Check sheet for the modelled part. Datum: model origin and axes. Units: mm. A direction names the side the tool comes from. Round coordinates to 2 decimals unless told otherwise and drop trailing zeros. Loops run counter-clockwise (first coordinate to the right, second up) from the corner with the lowest first, then second, coordinate; pieces in that order, holes last. Notation, with made-up numbers: (29, 54.25) -> (50, 54.25) arc R22 cw to (50, 77.25) -> close; hole circle Ø11 at (83.5, -28). An arc over 180 degrees is marked (long way). One line per item, written item: value. Start each with the question number.
1. Cross-section at C-C on z = 110. Record the cut outline in (x, y).
2. Go/stop test with flat-tipped pins: pin 1 (3 mm diameter, centred on x = -3, z = 37.5, fed in from +Y); pin 2 (8.5 mm diameter, centred on x = 2, z = 107.5, fed in from -Y); pin 3 (2 mm diameter, centred on x = -2, z = 102.5, fed in from +Y); pin 4 (13.5 mm diameter, centred on x = 0, y = 0, fed in from +Z). Record where each tip stops, or that it passes through.
3. Cross-section at A-A on y = 0. Record the cut outline in (x, z), then the cut area to 3 significant figures.
4. Release check for a two-part mould opening along Y. For faces 4 (the face through (12.114, 3.815, 108.46)), 5 (the face through (0, 11.5, 102)), 6 (the face through (2, -11.5, 108)), 7 (the face through (-2.395, -10.786, 108.46)) record: +Y half, -Y half, draft (parallel to the pull), parting line (faces both ways), or undercut.
5. Cross-section at D-D on x = -9. Record the cut outline in (y, z).
6. Material ranges on L1, parallel to Y at x = -0.25, z = 211; L2, parallel to Z at x = 0, y = -11.3; L3, parallel to X at y = 9.5, z = 85, recorded low to high.
7. Cross-section at B-B on x = 0. Record the cut outline in (y, z), then the cut area to 3 significant figures.
8. Set-up check for faces 1 (the face through (-1, -11.2, 0)), 2 (the face through (-6.494, 10.52, 110.286)), 3 (the face through (0, 11.5, 118)): record each of +Z, -Z, +X, -X, +Y, -Y from which the full face is reachable in a straight line by a thin tool's end or side.
from build123d import *

# Parameters (mm, degrees)
F0_R      = 12.7
F0_R_2    = 11.049
F1_DEPTH  = 220
F5_R      = 6.5
F6_DEPTH  = 15
F7_W      = 37.640377
F7_H      = 22
F8_DEPTH  = 1.2
F9_R      = 2.5
F10_DEPTH = 15
F11_W     = 50.336801
F11_H     = 16
F12_DEPTH = 1.2


with BuildPart() as f1:
    # F0 (on Top) → F1 (new body)
    with BuildSketch(Plane.XY):
        Circle(F0_R)
        Circle(F0_R_2, mode=Mode.SUBTRACT)
    extrude(amount=F1_DEPTH)

    # F5 (on offset) → F6 (cut)
    with BuildSketch(Plane.XZ.offset(-12.7)):
        with Locations((0, 110)):
            Circle(F5_R)
    extrude(amount=F6_DEPTH, mode=Mode.SUBTRACT)

    # F7 (on offset) → F8 (cut)
    with BuildSketch(Plane.XZ.offset(-12.7)):
        with Locations((-0.882831, 110)):
            Rectangle(F7_W, F7_H)
    extrude(amount=F8_DEPTH, mode=Mode.SUBTRACT)

    # F9 (on offset) → F10 (cut)
    with BuildSketch(Plane.XZ.offset(12.7)):
        with Locations((0, 110)):
            Circle(F9_R)
    extrude(amount=-F10_DEPTH, mode=Mode.SUBTRACT)

    # F11 (on offset) → F12 (cut)
    with BuildSketch(Plane.XZ.offset(12.7)):
        with Locations((-0.771954, 110)):
            Rectangle(F11_W, F11_H)
    extrude(amount=-F12_DEPTH, mode=Mode.SUBTRACT)


solid = f1.part
Taken from the geometry:
1. outline: (-6.5, 8.93) -> (-6.5, 10.91) arc R12.7 ccw to (-5.39, -11.5) -> (-2.5, -11.5) -> (-2.5, -10.76) arc R11.05 cw to start; (2.5, -11.5) -> (5.39, -11.5) arc R12.7 ccw to (6.5, 10.91) -> (6.5, 8.93) arc R11.05 cw to (2.5, -10.76) -> close
2. pin 1: stops at y = 12.61
2. pin 2: stops at y = -11.5
2. pin 3: stops at y = 11.5
2. pin 4: passes through
3. outline: (-12.7, 0) -> (-11.05, 0) -> (-11.05, 220) -> (-12.7, 220) -> close; (11.05, 0) -> (12.7, 0) -> (12.7, 220) -> (11.05, 220) -> close
3. area: 726 mm2
4. face 4: parting line
4. face 5: +Y half
4. face 6: -Y half
4. face 7: undercut
5. outline: (-8.96, 0) -> (-6.41, 0) -> (-6.41, 220) -> (-8.96, 220) -> close; (6.41, 0) -> (8.96, 0) -> (8.96, 220) -> (6.41, 220) -> close
6. L1: y = -12.7 to -11.05, 11.05 to 12.7
6. L2: z = 0 to 107.5, 112.5 to 220
6. L3: x = -8.43 to -5.64, 5.64 to 8.43
7. outline: (-12.7, 0) -> (-11.05, 0) -> (-11.05, 107.5) -> (-11.5, 107.5) -> (-11.5, 102) -> (-12.7, 102) -> close; (-12.7, 118) -> (-11.5, 118) -> (-11.5, 112.5) -> (-11.05, 112.5) -> (-11.05, 220) -> (-12.7, 220) -> close; (11.05, 0) -> (12.7, 0) -> (12.7, 99) -> (11.5, 99) -> (11.5, 103.5) -> (11.05, 103.5) -> close; (11.05, 116.5) -> (11.5, 116.5) -> (11.5, 121) -> (12.7, 121) -> (12.7, 220) -> (11.05, 220) -> close
7. area: 673 mm2
8. face 1: -Z, +X, -X, +Y, -Y
8. face 2: +Y
8. face 3: +X, -X, +Y
